Autodesk Inventor part; units mm, degrees
ref_plane "Work Plane1" through (0, 0, 0) normal (0, 0, 1) x (1, 0, 0)
ref_plane "YZ Plane" through (0, 0, 0) normal (1, 0, 0) x (0, 1, 0)
ref_plane "XZ Plane" through (0, 0, 0) normal (0, 1, 0) x (-1, 0, 0)
ref_plane "Work Plane1" through (0, 0, 0) normal (0, 0, 1) x (1, 0, 0)
sketch "Sketch1" plane through (0, 0, 0) normal (0, 0, 1) x (1, 0, 0)
  circle A0 centre (0, 0) radius 12
  circle A1 centre (-6.9282, -4) radius 2
  circle A2 centre (6.9282, -4) radius 2
  circle A3 centre (0, 8) radius 2
  line L0 (-4.8, 1) -> (-4.8, -1)
  line L1 (-3.873, 1) -> (-4.8, 1)
  arc A4 (-3.873, -1) -> (-3.873, 1) centre (0, 0) ccw
  line L2 (-4.8, -1) -> (-3.873, -1)
  point P0 (0, 0)
extrude "Extrusion1" add sketch "Sketch1" along normal blind 4 contours A0 | A1 | A2 | A3
sketch "Sketch2" plane through (0, 0, 0) normal (0, 0, -1) x (-1, 0, 0)
  point P0 (0, 0)
  point P1 (-6.9282, -4)
  point P2 (0, 8)
  point P3 (6.9282, -4)
hole "Hole1" at (6.9282, -4, 0) at (0, 8, 0) at (-6.9282, -4, 0) direction (0, 0, 1) diameter 4 end through all
properties part number "spiebaanplaatKlein" material "Aluminum 6061"
The model under review builds one solid part; all positions refer to its coordinate system, in mm. A direction names the side the tool comes from. Round coordinates to 2 decimals unless told otherwise and drop trailing zeros. Write each loop counter-clockwise with the first axis right and the second up, starting at its lowest first coordinate (ties: lowest second). Pieces come first, ordered by that corner, then holes.
(1) Wall thickness on L1, parallel to Y at x = 0, z = 1.5; L2, parallel to X at y = -3.5, z = 2.8; L3, parallel to Y at x = 0.5, z = 1: over which ranges is each line inside the solid? List them lowest first.
(2) We need section B-B on y = 3.5. Give the boundary of the cut face in (x, z), and give its area (3 significant figures).
(3) We need section A-A on x = 0. Give the boundary of the cut face in (y, z), and give its area (3 significant figures).
(4) We need section C-C on x = -4.25. Give the boundary of the cut face in (y, z).
(5) Mouldability with a two-part tool opening along Y and no side actions: class faces 3 (the cylindrical face through (-11.99, -0.53, 1.97)), 4 (the flat face through (-4.3, 1, 2)), 5 (the flat face through (-3, 3, 4)) as +Y half, -Y half, draft (parallel to the pull), parting line (faces both ways), or undercut.
(6) Machinability: for faces 1 (the flat face through (-3, 3, 0)), 2 (the flat face through (-4.3, -1, 2)), which of the approach directions +Z, -Z, +X, -X, +Y, -Y give a long, thin tool a straight path to every point of the face, cutting with its end or side? Answer none if there is none.
(7) Insertion check: pin 1 (0.5 mm diameter, centred on x = -4.5, z = 1, fed in from -Y); pin 2 (1 mm diameter, centred on x = -4.5, z = 1, fed in from +Y); pin 3 (2 mm diameter, centred on y = -4.5, z = 1.5, fed in from -X). Each pin has a flat end and moves straight along its axis. Give the tip position at first contact, or say it passes through.
(8) We need section D-D on y = -4.5. Give the boundary of the cut face in (x, z), and give its area (3 significant figures).
Findings below:
1. L1: y = -12 to -4, 4 to 6, 10 to 12
1. L2: x = -11.48 to -8.86, -4.99 to -1.94, 1.94 to 4.99, 8.86 to 11.48
1. L3: y = -11.99 to -3.97, 3.97 to 6.06, 9.94 to 11.99
2. outline: (-11.48, 0) - (-1.94, 0) - (-1.94, 4) - (-11.48, 4) - close; (1.94, 0) - (11.48, 0) - (11.48, 4) - (1.94, 4) - close
2. area: 76.3 mm2
3. outline: (-12, 0) - (-4, 0) - (-4, 4) - (-12, 4) - close; (4, 0) - (6, 0) - (6, 4) - (4, 4) - close; (10, 0) - (12, 0) - (12, 4) - (10, 4) - close
3. area: 48.0 mm2
4. outline: (-11.22, 0) - (-1, 0) - (-1, 4) - (-11.22, 4) - close; (1, 0) - (11.22, 0) - (11.22, 4) - (1, 4) - close
5. face 3: parting line
5. face 4: undercut
5. face 5: draft
6. face 1: -Z, +X, -X, +Y, -Y
6. face 2: +Z, -Z
7. pin 1: stops at y = -11.22
7. pin 2: stops at y = 11.31
7. pin 3: stops at x = -11.48
8. outline: (-11.12, 0) - (-8.86, 0) - (-8.86, 4) - (-11.12, 4) - close; (-4.99, 0) - (4.99, 0) - (4.99, 4) - (-4.99, 4) - close; (8.86, 0) - (11.12, 0) - (11.12, 4) - (8.86, 4) - close
8. area: 58.0 mm2
